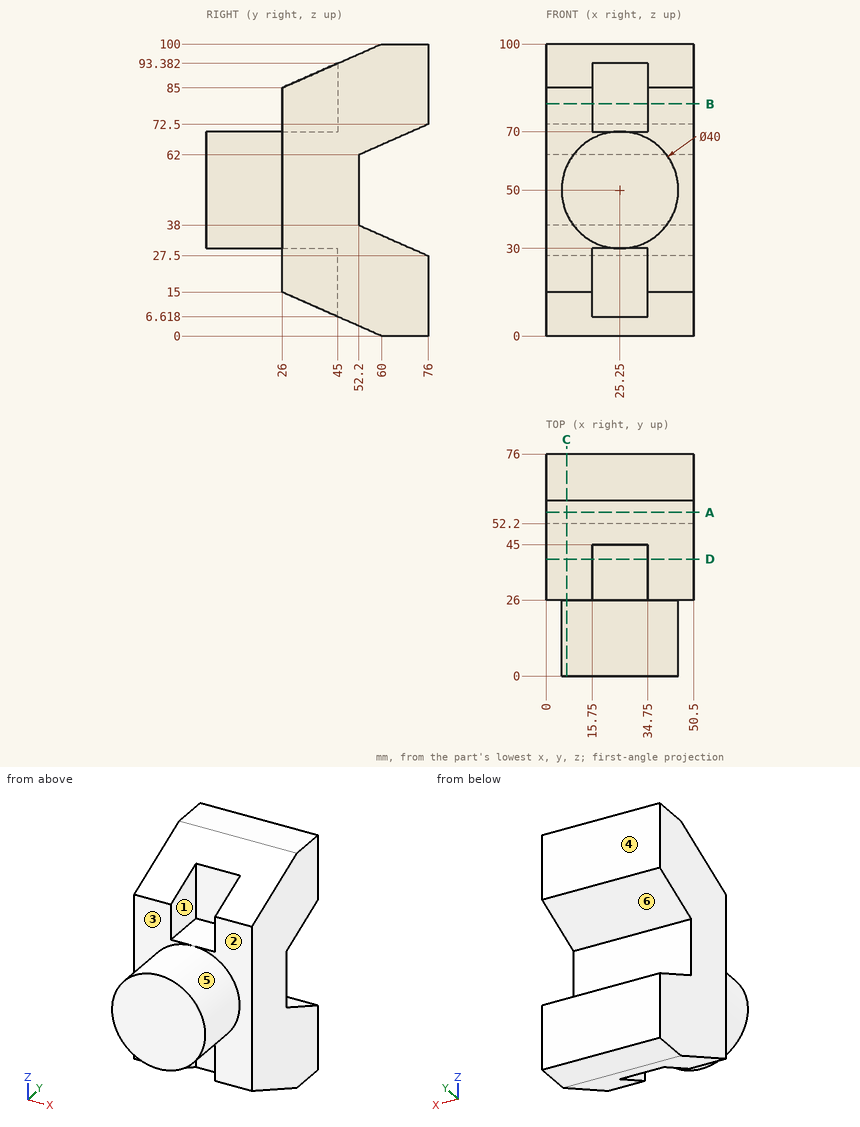
Geometry check sheet. Reference: drawing and pictorial views, mm from the part's lowest x, y, z. A direction names the side the tool comes from. Coordinates: 2 decimals unless noted, no trailing zeros. Write each loop counter-clockwise with the first axis right and the second up, starting at its lowest first coordinate (ties: lowest second). Pieces come first, ordered by that corner, then holes. Notation, with made-up numbers: (29, 46) -> (87, 46) arc R23 cw to (87, 75) -> close; hole circle Ø7 at (-34.5, 2.5). An arc over 180 degrees is marked (long way). Use a Markdown table: item, result.
1. Sectioned sample at D-D (y = 40). Enter the section's corners in (x, z), plus the area to 3 significant figures.
Reported:
| item | result |
|---|---|
| outline | (0, 8.82) -> (15.75, 8.82) -> (15.75, 30) -> (34.75, 30) -> (34.75, 8.82) -> (50.5, 8.82) -> (50.5, 91.18) -> (34.75, 91.18) -> (34.75, 70) -> (15.75, 70) -> (15.75, 91.18) -> (0, 91.18) -> close |
| area | 3,350 mm2 |
2. Release check for a two-part mould opening along Z. For the marked faces 4, 5 and 6 record: pulls with the +Z half, pulls with the -Z half, needs draft (parallel to the pull), parting line crosses it, or undercut.
Reported:
| item | result |
|---|---|
| face 4 | needs draft |
| face 5 | parting line crosses it |
| face 6 | undercut |
3. Tool access check on the marked faces 1, 2 and 3. Record the directions out of +Z, -Z, +X, -X, +Y, -Y that give a thin tool (end or side, any length) a straight path to the whole face; none if there is none.
Reported:
| item | result |
|---|---|
| face 1 | +Z, -Y |
| face 2 | +X, -Y |
| face 3 | -X, -Y |
4. Sectioned sample at C-C (x = 7). Enter the section's corners in (y, z).
Reported:
| item | result |
|---|---|
| outline | (0, 41.82) -> (26, 41.82) -> (26, 15) -> (60, 0) -> (76, 0) -> (76, 27.5) -> (52.2, 38) -> (52.2, 62) -> (76, 72.5) -> (76, 100) -> (60, 100) -> (26, 85) -> (26, 58.18) -> (0, 58.18) -> close |
5. Sectioned sample at A-A (y = 56). Enter the section's corners in (x, z) (1 decimal), plus the area to 3 significant figures.
Reported:
| item | result |
|---|---|
| outline | (0, 1.8) -> (50.5, 1.8) -> (50.5, 36.3) -> (0, 36.3) -> close; (0, 63.7) -> (50.5, 63.7) -> (50.5, 98.2) -> (0, 98.2) -> close |
| area | 3,490 mm2 |
6. Sectioned sample at B-B (z = 79.5). Enter the section's corners in (x, y), plus the area to 3 significant figures.
Reported:
| item | result |
|---|---|
| outline | (0, 26) -> (15.75, 26) -> (15.75, 45) -> (34.75, 45) -> (34.75, 26) -> (50.5, 26) -> (50.5, 76) -> (0, 76) -> close |
| area | 2,160 mm2 |
7. Scan lines: line 1 along Y through (x, z) = (40, 77.5); line 2 along Y through (x, z) = (22.5, 82); line 3 along Z through (x, y) = (32, 55) (1 decimal). Record each from-to range of solid material in increasing order.
Reported:
| item | result |
|---|---|
| line 1 | y = 26 to 76 |
| line 2 | y = 45 to 76 |
| line 3 | z = 2.2 to 36.8, 63.2 to 97.8 |
8. Go/stop test with flat-tipped pins: pin 1 Ø1.5 at (x, z) = (31.5, 43) entering from +Y; pin 2 Ø5 at (x, y) = (18, 26.5) entering from -Z; pin 3 Ø1 at (y, z) = (25, 31) entering from +X. Record where each tip stops, or that it passes through.
Reported:
| item | result |
|---|---|
| pin 1 | stops at y = 52.2 |
| pin 2 | stops at z = 14.3 |
| pin 3 | stops at x = 32.85 |
